```python
from build123d import *

# Parameters (mm, degrees)
SKETCH1_R           = 42.5
BOSS_EXTRUDE1_DEPTH = 2
SKETCH2_R           = 42.5
SKETCH2_R_2         = 41
BOSS_EXTRUDE2_DEPTH = 20
CHAMFER1_SIZE       = 2
CHAMFER2_SIZE       = 0.6


with BuildPart() as part:
    # Sketch1 → Boss-Extrude1 (new body)
    with BuildSketch(Plane(origin=(0, 0, 0), x_dir=(1, 0, 0), z_dir=(0, 1, 0))):
        with Locations(Location((0, 0, 0), (0, 0, 270))):
            Circle(SKETCH1_R)
    extrude(amount=BOSS_EXTRUDE1_DEPTH)

    # Sketch2 → Boss-Extrude2 (add)
    with BuildSketch(Plane(origin=(0, 2, 0), x_dir=(1, 0, 0), z_dir=(0, 1, 0))):
        with Locations(Location((0, 0, 0), (0, 0, 270))):
            Circle(SKETCH2_R)
        with Locations(Location((0, 0, 0), (0, 0, 270))):
            Circle(SKETCH2_R_2, mode=Mode.SUBTRACT)
    extrude(amount=BOSS_EXTRUDE2_DEPTH)

    # Chamfer1
    chamfer1_edges = [part.edges().sort_by_distance(p)[0] for p in [
        (0, 0, -42.5),
        (0, 2, -41),
    ]]
    chamfer(chamfer1_edges, length=CHAMFER1_SIZE)

    # Chamfer2
    chamfer2_edges = [part.edges().sort_by_distance(p)[0] for p in [
        (0, 22, -42.5),
    ]]
    chamfer(chamfer2_edges, length=CHAMFER2_SIZE)


solid = part.part
```
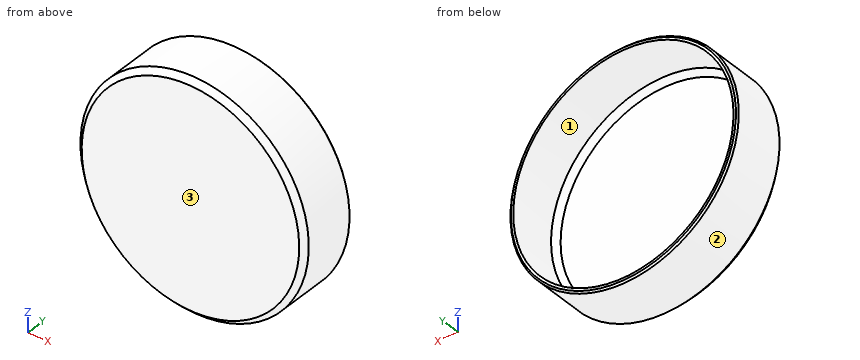
Geometry: final body of the model. Coordinates: model frame, mm. Face numbers are marked on the shaded views. Round coordinates to 2 decimals unless told otherwise and drop trailing zeros. Write each loop counter-clockwise with the first axis right and the second up, starting at its lowest first coordinate (ties: lowest second). Pieces come first, ordered by that corner, then holes. Notation, with made-up numbers: M 2.5,67 L 41.5,67 A31 cw 41.5,97 Z; hole C -30.5,-11 d2. An arc over 180 degrees is marked long. Answer in a Markdown table with one row per item. Add a question column.
(1) Cut plane A-A, the plane z = 0. Return the cut outline in (x, y), then the cut area to 3 significant figures.
(2) Cut plane C-C, the plane y = 16.75. Return the cut outline in (x, z).
(3) Ray query, L1, parallel to X at y = 9.5, z = 0; L2, parallel to Z at x = -1, y = 17; L3, parallel to Y at x = 22.5, z = 8. Return the intervals inside material, ascending.
(4) Contact query for flat-ended pins moving along their axis: pin 1 (2 mm diameter, centred on y = 14, z = 5.5, fed in from +X); pin 2 (3 mm diameter, centred on y = 4.5, z = 9, fed in from -X); pin 3 (2 mm diameter, centred on x = -23.5, y = 15, fed in from -Z). Output: stop coordinate, or through.
(5) Draft query along X for the marked faces 1, 2 and 3. Return one class per face: pulls with the +X half, pulls with the -X half, needs draft (parallel to the pull), parting line crosses it, or undercut.
(6) Cut plane B-B, the plane x = 0. Return the cut outline in (y, z), then the cut area to 3 significant figures.
Established:
| question | item | result |
|---|---|---|
| 1 | outline | M -42.5,2 L -40.5,0 L 40.5,0 L 42.5,2 L 42.5,21.4 L 41.9,22 L 41,22 L 41,4 L 39,2 L -39,2 L -41,4 L -41,22 L -41.9,22 L -42.5,21.4 Z |
| 1 | area | 230 mm² |
| 2 | outline | C 0,0 d85; hole C 0,0 d82 |
| 3 | L1 | -42.5 to -41, 41 to 42.5 |
| 3 | L2 | -42.49 to -40.99, 40.99 to 42.49 |
| 3 | L3 | 0 to 2 |
| 4 | pin 1 | x = 42.26 |
| 4 | pin 2 | x = -41.83 |
| 4 | pin 3 | z = -36.06 |
| 5 | face 1 | undercut |
| 5 | face 2 | parting line crosses it |
| 5 | face 3 | needs draft |
| 6 | outline | M 0,-40.5 L 2,-42.5 L 21.4,-42.5 L 22,-41.9 L 22,-41 L 4,-41 L 2,-39 L 2,39 L 4,41 L 22,41 L 22,41.9 L 21.4,42.5 L 2,42.5 L 0,40.5 Z |
| 6 | area | 230 mm² |
